For this review, take the finished solid that the model builds, in its own axes (mm). Face numbers are marked on the shaded views. A direction names the side the tool comes from. Round coordinates to 2 decimals unless told otherwise and drop trailing zeros. Order: outer loops, then holes, each group sorted by start corner. A loop starts at its lowest first (then second) coordinate and runs counter-clockwise, first axis right, second up.
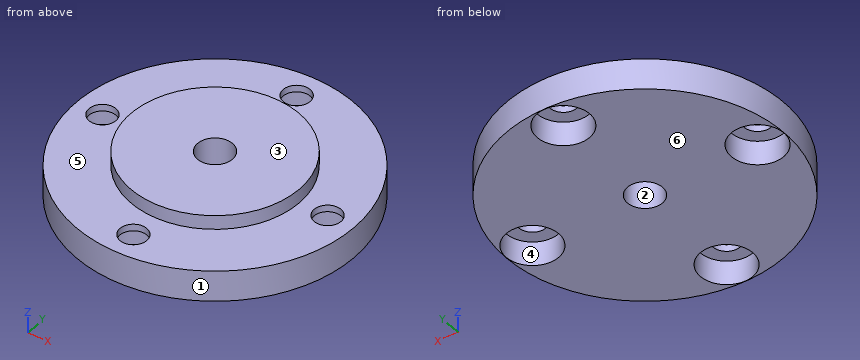
from build123d import *

# Parameters (mm, degrees)
SKETCH1_R                  = 12.573
BOSS_EXTRUDE1_DEPTH        = 2.794
SKETCH2_R                  = 7.62
BOSS_EXTRUDE2_DEPTH        = 1.27
CIRPATTERN2_COUNT          = 4
F_1_8_0_1250_DOWEL_HOLE2_D = 3.175


with BuildPart() as part:
    # Sketch1 → Boss-Extrude1 (new body)
    with BuildSketch(Plane.XY):
        Circle(SKETCH1_R)
    extrude(amount=BOSS_EXTRUDE1_DEPTH)

    # Sketch2 → Boss-Extrude2 (add)
    with BuildSketch(Plane.XY.offset(2.794)):
        Circle(SKETCH2_R)
    extrude(amount=BOSS_EXTRUDE2_DEPTH)

    # Sketch18 → CBORE for _2 Socket Head Cap Screw1 (revolve, cut)
    with BuildSketch(Plane.YZ.offset(-10.16)):
        Polygon((0, 0), (0, 8.446549267), (1.2192, 7.71398), (1.2192, 2.1844), (2.38125, 2.1844), (2.38125, 0), align=None)
    cbore_for_2_socket_head_cap_screw1 = revolve(axis=Axis((-10.16, 0, -6.35), (0, 0, 1)), mode=Mode.SUBTRACT)

    # CirPattern2: CBORE for _2 Socket Head Cap Screw1 ×4 about axis
    cirpattern2_axis = Axis((0, 0, 0), (0, 0, 1))
    for i in range(1, CIRPATTERN2_COUNT):
        add(cbore_for_2_socket_head_cap_screw1.rotate(cirpattern2_axis, i * 360 / CIRPATTERN2_COUNT), mode=Mode.SUBTRACT)

    # 1_8 _0.1250_ Dowel Hole2 (through all)
    with Locations(Plane(origin=(0, 0, 0), x_dir=(-1, 0, 0), z_dir=(0, 0, -1))):
        with Locations((0, 0)):
            Hole(F_1_8_0_1250_DOWEL_HOLE2_D / 2)


solid = part.part
(1) Clearance check with flat-ended pins moving along their axes: P1, Ø1.4, axis at x = -1, y = 10, coming from the -Z side; P2, Ø6, axis at x = 0, y = -2, coming from the -Z side; P3, Ø4.5, axis at x = 0, y = -10.16, coming from the +Z side. State where each tip first meets the part, or that it passes through.
(2) Draft analysis for pull direction Y (two halves, no side actions). For the marked faces 1, 2 and 3, state which applies: pulls with the +Y half, pulls with the -Y half, needs draft (parallel to the pull), parting line crosses it, or undercut.
(3) Add section C-C on y = 10.16. Give the boundary of the cut face in (x, z), plus the area to 3 significant figures.
(4) Tool access review of the marked faces 4, 5 and 6: name each direction out of +Z, -Z, +X, -X, +Y, -Y from which nothing blocks a thin tool from reaching the whole face with its end or side.
(5) Wall thickness on L1, parallel to X at y = -2, z = 1.5; L2, parallel to Z at x = 4, y = -8.5; L3, parallel to Y at x = 1.75, z = 1: over which ranges is each line inside the solid? List them lowest first.
(6) Add section A-A on x = 0. Count the separate pieces of the cut face and the enclosed holes in it, plus the area to 3 significant figures.
(7) Add section D-D on z = 3.15. Give the boundary of the cut face in (x, y) (1 decimal).
Here are the results:
1. P1: stops at z = 2.18
1. P2: stops at z = 0
1. P3: stops at z = 2.79
2. face 1: parting line crosses it
2. face 2: undercut
2. face 3: needs draft
3. outline: (-7.41, 0) - (-2.38, 0) - (-2.38, 2.18) - (-1.22, 2.18) - (-1.22, 2.79) - (-7.41, 2.79) - close; (1.22, 2.18) - (2.38, 2.18) - (2.38, 0) - (7.41, 0) - (7.41, 2.79) - (1.22, 2.79) - close
3. area: 29.5 mm2
4. face 4: -Z
4. face 5: +Z
4. face 6: -Z, +X, -X, +Y, -Y
5. L1: x = -12.41 to -11.45, -8.87 to 8.87, 11.45 to 12.41
5. L2: z = 0 to 2.79
5. L3: y = -12.45 to -11.77, -8.55 to 8.55, 11.77 to 12.45
6. separate pieces: 4
6. enclosed holes: 0
6. area: 52.9 mm2
7. outline: circle Ø15.2 at (0, 0); hole circle Ø3.2 at (0, 0)
